Build history of the part. All positions in model axes, mm. A direction names the side the tool comes from. Give positions to 0.01 mm unless a question says otherwise; leave off trailing zeros. Write each loop counter-clockwise with the first axis right and the second up, starting at its lowest first coordinate (ties: lowest second). Pieces come first, ordered by that corner, then holes.
from build123d import *

# Parameters (mm, degrees)
SKETCH_1_R             = 5
EXTRUDE_1_DEPTH        = 6
CUT_EXTRUDE_1_DEPTH    = 4
SKETCH_3_W             = 0.8
SKETCH_3_H             = 6.396892992
EXTRUDE_2_DEPTH        = 3
CHAMFER_1_SIZE         = 2
CHAMFER_1_SIZE2        = 0.352653961
CHAMFER_1_PART_2_SIZE  = 2
CHAMFER_1_PART_2_SIZE2 = 0.352653961


with BuildPart() as part:
    # Эскиз1 → Бобышка-Вытянуть1 (new body)
    with BuildSketch(Plane(origin=(0, 0, 0), x_dir=(1, 0, 0), z_dir=(0, 1, 0))):
        with Locations(Location((0, 0, 0), (0, 0, 270))):  # turned: the seam where the file's is
            Circle(SKETCH_1_R)
    extrude(amount=EXTRUDE_1_DEPTH)

    # Эскиз2 → Вырез-Вытянуть1 (cut)
    with BuildSketch(Plane(origin=(0, 6, 0), x_dir=(1, 0, 0), z_dir=(0, 1, 0))):
        with BuildLine():
            Line((-0.4, 3.198446496), (-0.4, -3.198446496))
            ThreePointArc((-0.4, -3.198446496), (-3.699699625, 0), (-0.4, 3.198446496))
        make_face()
        with BuildLine():
            Line((0.4, -3.198446496), (0.4, 3.198446496))
            ThreePointArc((0.4, 3.198446496), (3.699699625, 0), (0.4, -3.198446496))
        make_face()
    extrude(amount=-CUT_EXTRUDE_1_DEPTH, mode=Mode.SUBTRACT)

    # Эскиз3 → Бобышка-Вытянуть2 (add)
    with BuildSketch(Plane(origin=(0, 6, 0), x_dir=(1, 0, 0), z_dir=(0, 1, 0))):
        Rectangle(SKETCH_3_W, SKETCH_3_H)
    extrude(amount=EXTRUDE_2_DEPTH)

    # Фаска1
    chamfer_1_edges = [part.edges().sort_by_distance(p)[0] for p in [
        (0.4, 9, 0),
    ]]
    chamfer_1_side = [part.faces().sort_by_distance(p)[0] for p in [
        (0.4, 5.5, 0),
    ]]
    chamfer(chamfer_1_edges, length=CHAMFER_1_SIZE, length2=CHAMFER_1_SIZE2, reference=chamfer_1_side[0])

    # Фаска1 part 2
    chamfer_1_part_2_edges = [part.edges().sort_by_distance(p)[0] for p in [
        (-0.4, 9, 0),
    ]]
    chamfer_1_part_2_side = [part.faces().sort_by_distance(p)[0] for p in [
        (-0.4, 5.5, 0),
    ]]
    chamfer(chamfer_1_part_2_edges, length=CHAMFER_1_PART_2_SIZE, length2=CHAMFER_1_PART_2_SIZE2, reference=chamfer_1_part_2_side[0])


solid = part.part
1. Drill centre lines: line 1 along X through (y, z) = (5, 0.25); line 2 along Y through (x, z) = (2, 0.5); line 3 along X through (y, z) = (3, -0.75). Where is each one in solid material? Low to high.
2. Saw through at C-C on x = 3.25. Give the cut face in (y, z), plus the area to 3 significant figures.
3. Drop flat-ended pins along their axis: pin 1 (1 mm diameter, centred on x = -1.5, z = 0.5, fed in from +Y); pin 2 (0.9 mm diameter, centred on x = 0, y = 7.5, fed in from -Z); pin 3 (1.5 mm diameter, centred on x = -3.5, z = -3, fed in from -Y); pin 4 (6 mm diameter, centred on x = 3.5, z = -3, fed in from +Y). Give the stop position or say it passes through.
4. 3-axis set-ups, long thin cutter, end or side, ignore diameter. For faces 1 (the face through (2, 2, 0)), 2 (the face through (0.22, 8.01, 0.04)), 3 (the face through (0, 7, -3.198)): which of +Z, -Z, +X, -X, +Y, -Y reach the whole face in a straight line?
5. Saw through at D-D on y = 6.75. Give the cut face in (x, z), plus the area to 3 significant figures.
6. Saw through at B-B on z = 0. Give the cut face in (x, y), plus the area to 3 significant figures.
7. Mould opens along Z. For faces 4 (the face through (3.7, 4, -0.1)), 5 (the face through (0, 0, 0)), 6 (the face through (0, 7, 3.198)) say: pulls with the +Z half, pulls with the -Z half, needs draft (parallel to the pull), parting line crosses it, or undercut.
Outcome:
1. line 1: x = -4.99 to -3.69, -0.4 to 0.4, 3.69 to 4.99
1. line 2: y = 0 to 2
1. line 3: x = -4.94 to -3.61, -0.4 to 0.4, 3.61 to 4.94
2. outline: (0, -3.8) - (6, -3.8) - (6, -1.64) - (2, -1.64) - (2, 1.64) - (6, 1.64) - (6, 3.8) - (0, 3.8) - close
2. area: 32.5 mm2
3. pin 1: stops at y = 2
3. pin 2: stops at z = -3.2
3. pin 3: stops at y = 0
3. pin 4: stops at y = 6
4. face 1: +Y
4. face 2: +Z, -Z, +X, +Y
4. face 3: -Z, +X, -X, +Y
5. outline: (-0.4, -3.2) - (0.4, -3.2) - (0.4, 3.2) - (-0.4, 3.2) - close
5. area: 5.12 mm2
6. outline: (-5, 0) - (5, 0) - (5, 6) - (3.7, 6) - (3.7, 2) - (0.4, 2) - (0.4, 7) - (0.05, 9) - (-0.05, 9) - (-0.4, 7) - (-0.4, 2) - (-3.7, 2) - (-3.7, 6) - (-5, 6) - close
6. area: 35.3 mm2
7. face 4: undercut
7. face 5: needs draft
7. face 6: pulls with the +Z half
